Can you work these out from the drawing? Everything is in mm from the part's minimum corner. A direction names the side the tool comes from. Coordinates: 2 decimals unless noted, no trailing zeros. Write each loop counter-clockwise with the first axis right and the second up, starting at its lowest first coordinate (ties: lowest second). Pieces come first, ordered by that corner, then holes.
(1) For pin 1 Ø1 at (y, z) = (6.5, 2) entering from -X; pin 2 Ø4 at (y, z) = (7.5, 1.5) entering from -X (1 decimal); pin 3 Ø2 at (x, z) = (7, 1) entering from -Y, each with a flat end and sliding along its axis, tell me the tip position at first contact or that it passes through.
(2) Which directions (+Z, -Z, +X, -X, +Y, -Y) give clear straight access to the entire face, cutting with the end or side of a thin tool? Please do the marked faces 1 and 2.
(3) Imagine slicing it at D-D, the plane y = 15.5. List the corners of the cut face in (x, z) for me (1 decimal).
(4) Imagine slicing it at A-A, the plane z = 6.75. List the corners of the cut face in (x, y) for me.
(5) Imagine slicing it at B-B, the plane y = 5.5. List the corners of the cut face in (x, z) for me.
(6) Imagine slicing it at C-C, the plane z = 4.75. List the corners of the cut face in (x, y) for me (1 decimal).
(7) Please list where these lines run through material, in increasing order: probe 1 along Z at (x, y) = (3, 19.75); probe 2 along Y at (x, z) = (9.25, 3) (1 decimal); probe 3 along Y at (x, z) = (12.5, 2.5) (1 decimal).
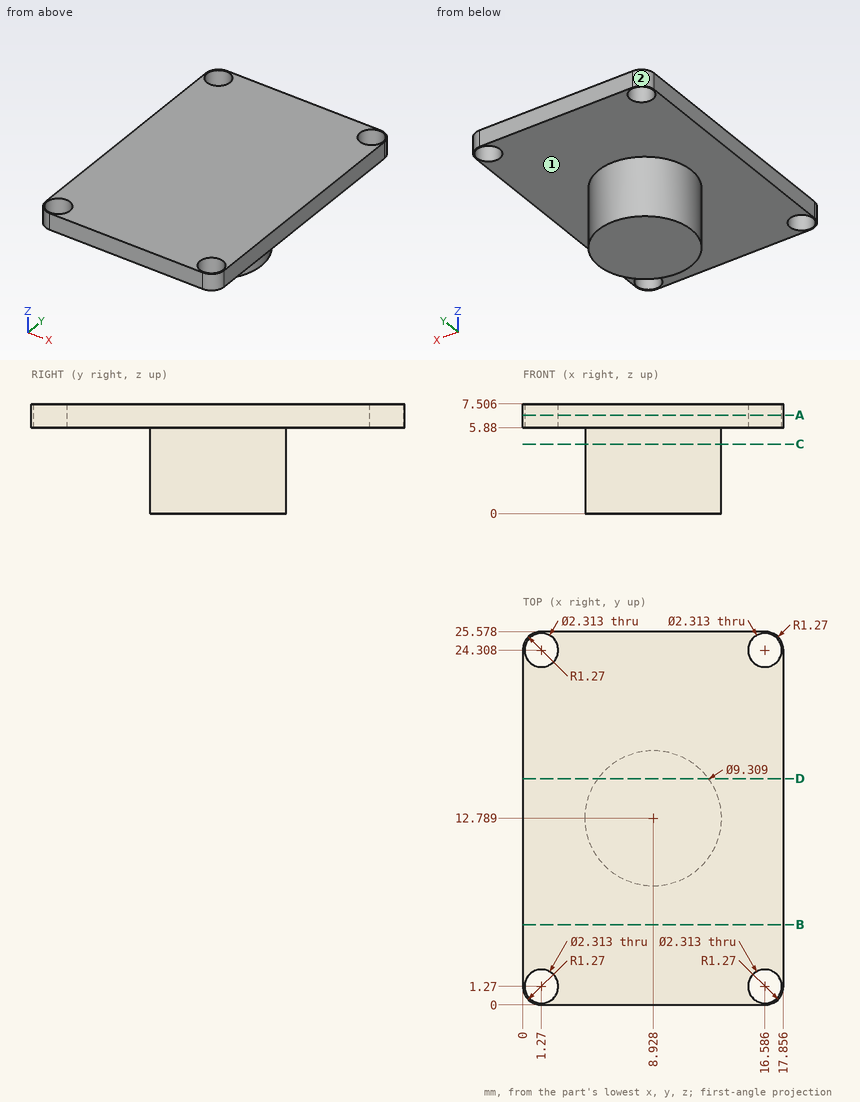
Recorded:
1. pin 1: passes through
1. pin 2: stops at x = 5.6
1. pin 3: stops at y = 8.23
2. face 1: -Z
2. face 2: +Z, -Z, -X, +Y
3. outline: (0, 5.9) - (5.1, 5.9) - (5.1, 0) - (12.7, 0) - (12.7, 5.9) - (17.9, 5.9) - (17.9, 7.5) - (0, 7.5) - close
4. outline: (0, 1.27) arc R1.27 ccw to (1.27, 0) - (16.59, 0) arc R1.27 ccw to (17.86, 1.27) - (17.86, 24.31) arc R1.27 ccw to (16.59, 25.58) - (1.27, 25.58) arc R1.27 ccw to (0, 24.31) - close; hole circle Ø2.31 at (1.27, 1.27); hole circle Ø2.31 at (1.27, 24.31); hole circle Ø2.31 at (16.59, 1.27); hole circle Ø2.31 at (16.59, 24.31)
5. outline: (0, 5.88) - (17.86, 5.88) - (17.86, 7.51) - (0, 7.51) - close
6. outline: circle Ø9.3 at (8.9, 12.8)
7. probe 1: z = 5.88 to 7.51
7. probe 2: y = 8.1 to 17.4
7. probe 3: y = 9.8 to 15.8
